Source: CAD feature listing. Evaluate the final solid. Frame: model axes, mm. A direction names the side the tool comes from. Coordinates: 2 decimals unless noted, no trailing zeros. Loops run counter-clockwise (first coordinate to the right, second up) from the corner with the lowest first, then second, coordinate; pieces in that order, holes last. Notation, with made-up numbers: (-33, 60) -> (-4, 60) arc R14 ccw to (-4, 76) -> close; hole circle Ø4 at (53.5, 2.5). An arc over 180 degrees is marked (long way). Answer as CSV lines item,"result".
from build123d import *

# Parameters (mm, degrees)
SKETCH1_W           = 100
SKETCH1_H           = 20
SKETCH1_R           = 2.15
BOSS_EXTRUDE1_DEPTH = 4
BOSS_EXTRUDE2_DEPTH = 7.5
FILLET1_R           = 8
FILLET2_R           = 3
FILLET3_R           = 20
SKETCH5_W           = 9.5
SKETCH5_H           = 20
SKETCH5_W_2         = 10.5
SKETCH5_W_3         = 7.5
BOSS_EXTRUDE3_DEPTH = 5
SKETCH6_W           = 3
SKETCH6_H           = 20
BOSS_EXTRUDE4_DEPTH = 26
BOSS_EXTRUDE5_DEPTH = 3
LPATTERN2_COUNT     = 2
LPATTERN2_PITCH     = 17
SKETCH9_R           = 1.15
CUT_EXTRUDE1_DEPTH  = 264.565931031
BOSS_EXTRUDE6_DEPTH = 20
FILLET4_R           = 2
CHAMFER1_SIZE       = 3
CHAMFER2_SIZE       = 5
FILLET5_R           = 2
FILLET6_R           = 2
BOSS_EXTRUDE7_DEPTH = 15
FILLET7_R           = 2


with BuildPart() as part:
    # Sketch1 → Boss-Extrude1 (new body)
    with BuildSketch(Plane.XY):
        with Locations((50, 10)):
            Rectangle(SKETCH1_W, SKETCH1_H)
        with Locations((70, 10)):
            Circle(SKETCH1_R, mode=Mode.SUBTRACT)
        with Locations(Location((30, 10, 0), (0, 0, 180))):
            Circle(SKETCH1_R, mode=Mode.SUBTRACT)
        with Locations((10, 10)):
            Circle(SKETCH1_R, mode=Mode.SUBTRACT)
        with Locations(Location((90, 10, 0), (0, 0, 180))):
            Circle(SKETCH1_R, mode=Mode.SUBTRACT)
    extrude(amount=BOSS_EXTRUDE1_DEPTH)

    # Fillet6
    fillet6_edges = [part.edges().sort_by_distance(p)[0] for p in [
        (0, 20, 2),
        (100, 20, 2),
        (100, 0, 2),
        (0, 0, 2),
    ]]
    fillet(fillet6_edges, radius=FILLET6_R)



with BuildPart() as body_2:
    # Sketch4 → Boss-Extrude2 (new, symmetric)
    with BuildSketch(Plane.ZY.offset(-50)):
        Polygon((0, 2.5), (0, 17.5), (-1, 17.5), (-193, 123.393201871), (-193, 155), (-201, 155), (-201, 56.089838486), (-1, 2.5), align=None)
        Polygon((-41.271401161, 28.290689419), (-193, 68.946244947), (-193, 111.973122473), align=None, mode=Mode.SUBTRACT)
    extrude(amount=BOSS_EXTRUDE2_DEPTH, both=True)

    # Fillet1
    fillet1_edges = [body_2.edges().sort_by_distance(p)[0] for p in [
        (50, 111.973122473, -193),
        (50, 68.946244947, -193),
    ]]
    fillet(fillet1_edges, radius=FILLET1_R)

    # Fillet2
    fillet2_edges = [body_2.edges().sort_by_distance(p)[0] for p in [
        (50, 28.290689419, -41.271401161),
    ]]
    fillet(fillet2_edges, radius=FILLET2_R)

    # Fillet3
    fillet3_edges = [body_2.edges().sort_by_distance(p)[0] for p in [
        (50, 56.089838486, -201),
    ]]
    fillet(fillet3_edges, radius=FILLET3_R)

    # Sketch5 → Boss-Extrude3 (add, symmetric)
    with BuildSketch(Plane.XY.offset(-193)):
        with Locations((27.25, 145)):
            Rectangle(SKETCH5_W, SKETCH5_H)
        with Locations((37.25, 145)):
            Rectangle(SKETCH5_W_2, SKETCH5_H)
        with Locations((46.25, 145)):
            Rectangle(SKETCH5_W_3, SKETCH5_H)
        with Locations((53.75, 145)):
            Rectangle(SKETCH5_W_3, SKETCH5_H)
        with Locations((62.75, 145)):
            Rectangle(SKETCH5_W_2, SKETCH5_H)
        with Locations((72.75, 145)):
            Rectangle(SKETCH5_W, SKETCH5_H)
    extrude(amount=BOSS_EXTRUDE3_DEPTH, both=True)

    # Sketch6 → Boss-Extrude4 (add)
    with BuildSketch(Plane.XY.offset(-188)):
        with Locations((30.5, 145)):
            Rectangle(SKETCH6_W, SKETCH6_H)
        with Locations((69.5, 145)):
            Rectangle(SKETCH6_W, SKETCH6_H)
    extrude(amount=BOSS_EXTRUDE4_DEPTH)

    # Sketch8 → Boss-Extrude5 (add)
    with BuildSketch(Plane(origin=(0, 155, 0), x_dir=(1, 0, 0), z_dir=(0, 1, 0))):
        Polygon((22.5, 188), (29, 162), (29, 174), (25.5, 188), align=None)
        Polygon((74.5, 188), (77.5, 188), (71, 162), (71, 174), align=None)
    boss_extrude5 = extrude(amount=-BOSS_EXTRUDE5_DEPTH)

    # LPattern2: Boss-Extrude5 ×2
    with Locations(*[(0, -i * LPATTERN2_PITCH, 0) for i in range(1, LPATTERN2_COUNT)]):
        add(boss_extrude5)

    # Sketch9 → Cut-Extrude1 (cut, through all)
    with BuildSketch(Plane(origin=(71, 0, 0), x_dir=(0, 0, -1), z_dir=(1, 0, 0))):
        with Locations((164.6, 145)):
            Circle(SKETCH9_R)
    extrude(amount=-CUT_EXTRUDE1_DEPTH, mode=Mode.SUBTRACT)

    # Sketch10 → Boss-Extrude6 (add)
    with BuildSketch(Plane(origin=(0, 155, 0), x_dir=(1, 0, 0), z_dir=(0, 1, 0))):
        Polygon((57.5, 201), (57.5, 198), (77.5, 198), align=None)
        Polygon((42.5, 201), (42.5, 198), (22.5, 198), align=None)
    extrude(amount=-BOSS_EXTRUDE6_DEPTH)

    # Fillet4
    fillet4_edges = [body_2.edges().sort_by_distance(p)[0] for p in [
        (32, 145, -188),
        (68, 145, -188),
        (77.5, 145, -198),
        (22.5, 145, -198),
    ]]
    fillet(fillet4_edges, radius=FILLET4_R)

    # Chamfer1
    chamfer1_edges = [body_2.edges().sort_by_distance(p)[0] for p in [
        (50, 135, -193),
    ]]
    chamfer(chamfer1_edges, length=CHAMFER1_SIZE)

    # Chamfer2
    # the kernel refuses this chamfer: 5 mm, written as the material it adds along each edge
    with BuildSketch(Plane(origin=(57.5, 135, -177.14158506), x_dir=(0.9996219169112968, 0.0274958766105877, 0), z_dir=(0, 0, -1))) as chamfer2_piece_1_section:
        Polygon((CHAMFER2_SIZE * 0.999621916911, CHAMFER2_SIZE * 0.0274958766106), (-CHAMFER2_SIZE * 0.0274958766106, CHAMFER2_SIZE * 0.999621916911), (0, 0), align=None)
    chamfer2_piece_1 = extrude(amount=23.85841494, mode=Mode.PRIVATE)
    chamfer2_piece_1 = split(chamfer2_piece_1, bisect_by=Plane(origin=(57.857106813, 131.163616626, -193.836383374), z_dir=(0, -0.7071067811865476, 0.7071067811865476)), keep=Keep.TOP, mode=Mode.PRIVATE)
    chamfer2_piece_1 = split(chamfer2_piece_1, bisect_by=Plane(origin=(57.857106813, 130.884822168, -193), z_dir=(0, 0, -1)), keep=Keep.TOP, mode=Mode.PRIVATE)
    add(chamfer2_piece_1)
    with BuildSketch(Plane(origin=(57.5, 135, -177.14158506), x_dir=(0.9996219169112968, 0.0274958766105877, 0), z_dir=(0, 0, -1))) as chamfer2_piece_2_section:
        Polygon((CHAMFER2_SIZE * 0.999621916911, CHAMFER2_SIZE * 0.0274958766106), (-CHAMFER2_SIZE * 0.0274958766106, CHAMFER2_SIZE * 0.999621916911), (0, 0), align=None)
    chamfer2_piece_2 = extrude(amount=23.85841494, mode=Mode.PRIVATE)
    chamfer2_piece_2 = split(chamfer2_piece_2, bisect_by=Plane(origin=(59.611963913, 133.659604806, -191.340395194), z_dir=(0, 0.7071067811865476, -0.7071067811865476)), keep=Keep.TOP, mode=Mode.PRIVATE)
    chamfer2_piece_2 = split(chamfer2_piece_2, bisect_by=Plane(origin=(59.611963913, 134.212806408, -193), z_dir=(0, 0, 1)), keep=Keep.TOP, mode=Mode.PRIVATE)
    add(chamfer2_piece_2)
    with BuildSketch(Plane(origin=(57.5, 135, -177.14158506), x_dir=(0.9996219169112968, 0.0274958766105877, 0), z_dir=(0, 0, -1))) as chamfer2_piece_3_section:
        Polygon((CHAMFER2_SIZE * 0.999621916911, CHAMFER2_SIZE * 0.0274958766106), (-CHAMFER2_SIZE * 0.0274958766106, CHAMFER2_SIZE * 0.999621916911), (0, 0), align=None)
    chamfer2_piece_3 = extrude(amount=23.85841494, mode=Mode.PRIVATE)
    chamfer2_piece_3 = split(chamfer2_piece_3, bisect_by=Plane(origin=(59.139397436, 130.720913617, -194.279086383), z_dir=(0, 0.7071067811865476, -0.7071067811865476)), keep=Keep.TOP, mode=Mode.PRIVATE)
    chamfer2_piece_3 = split(chamfer2_piece_3, bisect_by=Plane(origin=(59.699836307, 133.375592649, -200.670024554), z_dir=(-0.14834045293024603, 0, 0.9889363528682974)), keep=Keep.TOP, mode=Mode.PRIVATE)
    chamfer2_piece_3 = split(chamfer2_piece_3, bisect_by=Plane(origin=(59.139397436, 133.375592649, -193), z_dir=(0, 0, -1)), keep=Keep.TOP, mode=Mode.PRIVATE)
    add(chamfer2_piece_3)
    with BuildSketch(Plane(origin=(42.5, 135, -201), x_dir=(-0.9996219169112968, 0.0274958766105877, 0), z_dir=(0, 0, 1))) as chamfer2_piece_4_section:
        Polygon((CHAMFER2_SIZE * 0.999621916911, CHAMFER2_SIZE * 0.0274958766106), (-CHAMFER2_SIZE * 0.0274958766106, CHAMFER2_SIZE * 0.999621916911), (0, 0), align=None)
    chamfer2_piece_4 = extrude(amount=23.85841494, mode=Mode.PRIVATE)
    chamfer2_piece_4 = split(chamfer2_piece_4, bisect_by=Plane(origin=(40.860602564, 130.720913617, -194.279086383), z_dir=(0, 0.7071067811865476, -0.7071067811865476)), keep=Keep.TOP, mode=Mode.PRIVATE)
    chamfer2_piece_4 = split(chamfer2_piece_4, bisect_by=Plane(origin=(40.300163693, 133.375592649, -200.670024554), z_dir=(0.1483404529302461, 0, 0.9889363528682974)), keep=Keep.TOP, mode=Mode.PRIVATE)
    chamfer2_piece_4 = split(chamfer2_piece_4, bisect_by=Plane(origin=(40.860602564, 133.375592649, -193), z_dir=(0, 0, -1)), keep=Keep.TOP, mode=Mode.PRIVATE)
    add(chamfer2_piece_4)
    with BuildSketch(Plane(origin=(42.5, 135, -201), x_dir=(-0.9996219169112968, 0.0274958766105877, 0), z_dir=(0, 0, 1))) as chamfer2_piece_5_section:
        Polygon((CHAMFER2_SIZE * 0.999621916911, CHAMFER2_SIZE * 0.0274958766106), (-CHAMFER2_SIZE * 0.0274958766106, CHAMFER2_SIZE * 0.999621916911), (0, 0), align=None)
    chamfer2_piece_5 = extrude(amount=23.85841494, mode=Mode.PRIVATE)
    chamfer2_piece_5 = split(chamfer2_piece_5, bisect_by=Plane(origin=(42.142893187, 131.163616626, -193.836383374), z_dir=(0, -0.7071067811865476, 0.7071067811865476)), keep=Keep.TOP, mode=Mode.PRIVATE)
    chamfer2_piece_5 = split(chamfer2_piece_5, bisect_by=Plane(origin=(42.142893187, 130.884822168, -193), z_dir=(0, 0, -1)), keep=Keep.TOP, mode=Mode.PRIVATE)
    add(chamfer2_piece_5)
    with BuildSketch(Plane(origin=(42.5, 135, -201), x_dir=(-0.9996219169112968, 0.0274958766105877, 0), z_dir=(0, 0, 1))) as chamfer2_piece_6_section:
        Polygon((CHAMFER2_SIZE * 0.999621916911, CHAMFER2_SIZE * 0.0274958766106), (-CHAMFER2_SIZE * 0.0274958766106, CHAMFER2_SIZE * 0.999621916911), (0, 0), align=None)
    chamfer2_piece_6 = extrude(amount=23.85841494, mode=Mode.PRIVATE)
    chamfer2_piece_6 = split(chamfer2_piece_6, bisect_by=Plane(origin=(40.388036087, 133.659604806, -191.340395194), z_dir=(0, 0.7071067811865476, -0.7071067811865476)), keep=Keep.TOP, mode=Mode.PRIVATE)
    chamfer2_piece_6 = split(chamfer2_piece_6, bisect_by=Plane(origin=(40.388036087, 134.212806408, -193), z_dir=(0, 0, 1)), keep=Keep.TOP, mode=Mode.PRIVATE)
    add(chamfer2_piece_6)

    # Fillet5
    fillet5_edges = [body_2.edges().sort_by_distance(p)[0] for p in [
        (30.5, 155, -162),
        (30.5, 135, -162),
        (69.5, 155, -162),
        (69.5, 135, -162),
    ]]
    fillet(fillet5_edges, radius=FILLET5_R)


with BuildPart() as part_1:
    add(part.part)

    add(body_2.part)  # Boss-Extrude7 merges body 2
    # Sketch11 → Boss-Extrude7 (add)
    with BuildSketch(Plane(origin=(0, 17.5, 0), x_dir=(1, 0, 0), z_dir=(0, 1, 0))):
        Polygon((57.5, 1), (57.5, 0), (66.5, 0), align=None)
        Polygon((42.5, 1), (42.5, 0), (33.5, 0), align=None)
    extrude(amount=-BOSS_EXTRUDE7_DEPTH)

    # Fillet7
    fillet7_edges = [part_1.edges().sort_by_distance(p)[0] for p in [
        (57.5, 70.446600935, -97),
        (42.5, 70.446600935, -97),
    ]]
    fillet(fillet7_edges, radius=FILLET7_R)


solid = part_1.part
(1) Pin query (flat end, axial travel): pin 1 Ø6.5 at (y, z) = (141, -192.5) entering from +X; pin 2 Ø2.5 at (x, y) = (30, 146.5) entering from +Z; pin 3 Ø8 at (x, z) = (40, -146.5) entering from +Y; pin 4 Ø12 at (x, z) = (36, -53.5) entering from +Y. Return the tip coordinate at first contact, or that it passes through.
Computed values:
pin 1,"x = 77.5"
pin 2,"z = -162"
pin 3,"y = 98.54"
pin 4,"through"
(2) Access query for faces 4 (the flat face through (32, 145, -174)), 5 (the flat face through (50, 87, -193)), 6 (the flat face through (29, 145, -175)), 7 (the flat face through (73, 152, -178)), 8 (the flat face through (42.5, 48, -116)). Directions: +Z, -Z, +X, -X, +Y, -Y. A direction counts if a zero-diameter tool reaches every point of the face in a straight line with its end or side. Return the directions, or none.
Computed values:
face 4,"+Z, +Y, -Y"
face 5,"+X, -X"
face 6,"none"
face 7,"+Z, +X"
face 8,"-Z, -X, -Y"
(3) Material intervals for L1, parallel to Y at x = 70, z = 2.55; L2, parallel to Z at x = 51.5, y = 72; L3, parallel to Z at x = 30.7, y = 145, sorted ascending. Write a range as [from, to].
Computed values:
L1,"[0, 7.85], [12.15, 20]"
L2,"[-201, -192.38], [-120.52, -99.82]"
L3,"[-199.23, -165.75], [-163.45, -162]"
(4) Cut plane A-A (x = 48.5). Return the cut outline in (y, z).
Computed values:
outline,"(0, 0) -> (2.5, 0) -> (2.5, -1) -> (52.12, -186.18) arc R20 ccw to (71.44, -201) -> (155, -201) -> (155, -188) -> (135, -188) -> (135, -190) -> (132, -193) -> (123.39, -193) -> (17.5, -1) -> (17.5, 0) -> (20, 0) -> (20, 4) -> (0, 4) -> close; hole (34.67, -65.08) -> (67.36, -187.07) arc R8 ccw to (75.08, -193) -> (98.42, -193) arc R8 ccw to (105.43, -181.14) -> (40.2, -62.86) arc R3 ccw to start"
(5) Draft query along Z for faces 1 (the cylindrical face through (50.105, 70.157, -191.302)), 2 (the flat face through (22.5, 145, -192)), 3 (the cylindrical face through (50.105, 59.116, -196.755)). Return one class per face: released by +Z, released by -Z, zero draft, split by the parting line, or undercut.
Computed values:
face 1,"undercut"
face 2,"zero draft"
face 3,"released by -Z"
